Here's how the part is built. I have some questions about the finished solid (model axes, mm). A direction names the side the tool comes from. Round coordinates to 2 decimals unless told otherwise and drop trailing zeros. Write each loop counter-clockwise with the first axis right and the second up, starting at its lowest first coordinate (ties: lowest second). Pieces come first, ordered by that corner, then holes. Notation, with made-up numbers: (40.5, -19) -> (68.5, -19) arc R10 ccw to (68.5, -13) -> close; hole circle Ø8 at (52.25, -36.5). An arc over 180 degrees is marked (long way). Answer as CSV lines item,"result".
Autodesk Inventor part; units mm, degrees
ref_plane "YZ Plane" through (0, 0, 0) normal (1, 0, 0) x (0, 1, 0)
ref_plane "XZ Plane" through (0, 0, 0) normal (0, 1, 0) x (-1, 0, 0)
ref_plane "XY Plane" through (0, 0, 0) normal (0, 0, 1) x (1, 0, 0)
sketch "Sketch1" plane through (0, 0, 0) normal (0, 1, 0) x (-1, 0, 0)
  line L0 (45, 0) -> (45, -45)
  line L1 (45, -45) -> (0, -45)
  line L2 (-45, 0) -> (-45, -45)
  line L3 (-45, -45) -> (0, -45)
  line L4 (45, 0) -> (45, 45)
  line L5 (45, 45) -> (0, 45)
  line L6 (-45, 0) -> (-45, 45)
  line L7 (-45, 45) -> (0, 45)
  line L8 (-45, 45) -> (-45, 35)
  line L9 (-45, 35) -> (51.6203, 35)
  line L10 (-45, -45) -> (-45, -35)
  line L11 (-45, -35) -> (58.872, -35)
  line L12 (45, 45) -> (35, 45)
  line L13 (35, 45) -> (35, -45)
  point P0 (0, 0)
  point P1 (35, 35)
  point P2 (35, -35)
  dimension "d0" = 45
  dimension "d1" = 45
  dimension "d2" = 10
  dimension "d3" = 10
  dimension "d4" = 10
extrude "Extrusion1" add sketch "Sketch1" along normal blind 60 contours L0 L11 L13 L9 L4 | L0 L1 L13 L11 | L9 L13 L5 L4 | L13 L1 L3 L2 L11 | L9 L6 L7 L5 L13
fillet "Fillet1" radius 20 2 edges at (-35, 30, 35) (-35, 30, -35)
fillet "Fillet2" radius 5 2 edges at (-45, 30, 45) (-45, 30, -45)
sketch "Sketch2" plane through (45, 0, -45) normal (0, 0, -1) x (-1, 0, 0)
  line L0 (0, 0) -> (0, 60)
  arc A0 (46.5831, 55) -> (46.5831, 5) centre (30, 30) ccw
  line L1 (90, 5) -> (46.5831, 5)
  line L2 (46.5831, 55) -> (90, 55)
  line L3 (90, 60) -> (90, 0)
  line L4 (60, 0) -> (0, 0)
  line L5 (90, 60) -> (0, 60)
  line L6 (0, 60) -> (0, 0)
  line L7 (0, 0) -> (90, 0)
  line L8 (90, 0) -> (90, 60)
  point P0 (45, 0)
  point P1 (30, 60)
  point P2 (30, 0)
  point P3 (0, 30)
  dimension "d10" = 5
extrude "Extrusion2" cut sketch "Sketch2" against normal blind 161.25 contours L0 A0 L4 | L0 L5 A0 | A0 L1 L3 L7 L4 | L5 L3 L2 A0
sketch "Sketch3" plane through (-1.5831, 5, -45) normal (0, 0, -1) x (-1, 0, 0)
  line L0 (13.4169, 50) -> (0, 50)
  arc A0 (0, 50) -> (0, 0) centre (-16.5831, 25) ccw
  circle A1 centre (-16.5831, 25) radius 2.5
  point P0 (-1.5831, -5)
  dimension "d15" = 5
extrude "Extrusion3" cut sketch "Sketch3" against normal blind 161.25
sketch "Sketch4" plane through (-45, 5, 40) normal (-1, 0, 0) x (0, 0, 1)
  circle A0 centre (-40, 25) radius 2.5
  point P0 (-40, -5)
  dimension "d18" = 5
extrude "Extrusion4" cut sketch "Sketch4" against normal blind 161.25
sketch "Sketch5" plane through (-45, 5, 40) normal (-1, 0, 0) x (0, 0, 1)
  point P0 (-40, -5)
sketch "Sketch6" plane through (-35, 5, -15) normal (1, 0, 0) x (0, 0, -1)
  line L0 (-15, 45) -> (-5, 45)
  line L1 (-5, 45) -> (-5, 5)
  line L2 (-5, 5) -> (-25, 5)
  line L3 (-25, 5) -> (-25, 45)
  line L4 (-25, 45) -> (-15, 45)
  point P0 (-15, -5)
  point P1 (-15, 25)
  dimension "d21" = 20
  dimension "d22" = 10
  dimension "d23" = 40
  dimension "d24" = 20
  dimension "d25" = 40
  dimension "d26" = 90
extrude "Extrusion5" cut sketch "Sketch6" against normal blind 5
properties part number "PartArm1"
1. Suppose I cut it at C-C on z = 0. Please give me the cut outline in (x, y).
Numbers:
outline,"(-45, 5) -> (-35, 5) -> (-35, 10) -> (-40, 10) -> (-40, 27.5) -> (-45, 27.5) -> close; (-45, 32.5) -> (-40, 32.5) -> (-40, 50) -> (-35, 50) -> (-35, 55) -> (-45, 55) -> close"
2. Suppose I cut it at D-D on z = 36.5. Please give me the cut outline in (x, y), and give its area (3 significant figures).
Numbers:
outline,"(-45, 5) -> (-1.58, 5) arc R30 ccw (long way) to (-1.58, 55) -> (-45, 55) -> close; hole circle Ø5 at (15, 30)"
area,"4,510 mm^2"
3. Suppose I cut it at A-A on x = -4. Please give me the cut outline in (y, z), and give its area (3 significant figures).
Numbers:
outline,"(5, -45) -> (55, -45) -> (55, -35) -> (5, -35) -> close; (5, 35) -> (55, 35) -> (55, 45) -> (5, 45) -> close"
area,"1,000 mm^2"
4. For pin 1 Ø6 at (x, z) = (-36, 11) entering from +Y; pin 2 Ø1 at (y, z) = (13, -20.5) entering from +X; pin 3 Ø1.5 at (y, z) = (31, -2) entering from +X; pin 4 Ø6 at (x, y) = (15, 30) entering from -Z, each with a flat end and sliding along its axis, tell me the tip position at first contact or that it passes through.
Numbers:
pin 1,"stops at y = 55"
pin 2,"stops at x = -34.08"
pin 3,"stops at x = -40"
pin 4,"stops at z = -45"
5. If I drill on line 1 (Z direction, x = 5, y = 19.5); line 2 (Y direction, x = -43.8, z = 0); line 3 (Y direction, x = 15, z = 38), over which ranges is the centre line in solid material (lowest first)?
Numbers:
line 1,"z = -45 to -35, 35 to 45"
line 2,"y = 5 to 27.5, 32.5 to 55"
line 3,"y = 0 to 27.5, 32.5 to 60"
6. If we mould it in two halves opening along Y, with no side actions, what happens to faces 1 (the face through (-37, 30, 10)), 2 (the face through (2, 30, 45)), 3 (the face through (-37, 50, 0)), 4 (the face through (-37, 55, -1))? For each: released by +Y, released by -Y, zero draft, split by the parting line, or undercut.
Numbers:
face 1,"undercut"
face 2,"zero draft"
face 3,"undercut"
face 4,"released by +Y"
7. Suppose I cut it at B-B on y = 30. Please give me the cut outline in (x, z).
Numbers:
outline,"(-45, -40) arc R5 ccw to (-40, -45) -> (12.5, -45) -> (12.5, -35) -> (-15, -35) arc R20 cw to (-35, -15) -> (-35, -10) -> (-40, -10) -> (-40, -2.5) -> (-45, -2.5) -> close; (-45, 2.5) -> (-40, 2.5) -> (-40, 10) -> (-35, 10) -> (-35, 15) arc R20 cw to (-15, 35) -> (12.5, 35) -> (12.5, 45) -> (-40, 45) arc R5 ccw to (-45, 40) -> close; (17.5, -45) -> (45, -45) -> (45, -35) -> (17.5, -35) -> close; (17.5, 35) -> (45, 35) -> (45, 45) -> (17.5, 45) -> close"
8. On a 3-axis mill with a long thin cutter (end or side, diameter ignored), from which of +Z, -Z, +X, -X, +Y, -Y can I reach the whole of each face in a straight line? I mean faces 5 (the face through (-38, 5, -1)), 6 (the face through (-40, 30, -4)), 7 (the face through (-29.297, 30.35, 28.986)), 8 (the face through (-43, 30, -44)). Say none if no direction works.
Numbers:
face 5,"+Z, -Z, -X, -Y"
face 6,"+X"
face 7,"+X, +Y, -Y"
face 8,"-Z, -X, +Y, -Y"
